```python
from build123d import *

# Parameters (mm, degrees)
SKETCH_R     = 3.375
PAD_DEPTH    = 3
SKETCH001_R  = 3.375
PAD001_DEPTH = 3
PAD002_DEPTH = 3
PAD003_DEPTH = 3
PAD004_DEPTH = 3


with BuildPart() as part:
    # Sketch → Pad (new body)
    with BuildSketch(Plane.XZ):
        with BuildLine():
            Line((-12.7, 0), (12.7, 0))
            Line((12.7, 0), (12.7, 52))
            ThreePointArc((12.7, 52), (0, 57.173882), (-12.7, 52))
            Line((-12.7, 52), (-12.7, 0))
        make_face()
        with Locations((0, 39)):
            Circle(SKETCH_R, mode=Mode.SUBTRACT)
        with Locations((0, 13)):
            Circle(SKETCH_R, mode=Mode.SUBTRACT)
    extrude(amount=-PAD_DEPTH)

    # Sketch001 → Pad001 (join)
    with BuildSketch(Plane.XY):
        with BuildLine():
            Line((-56.33961, 0), (-86.996465, 30.656854))
            ThreePointArc((-55.176659, 62.476659), (-78.231159, 53.711354), (-86.996465, 30.656854))
            Line((-55.176659, 62.476659), (4.3, 3))
            Line((4.3, 3), (-12.7, 3))
            Line((-12.7, 3), (-12.7, 0))
            Line((-56.33961, 0), (-12.7, 0))
        make_face()
        with Locations((-56.944426, 32.424621)):
            Circle(SKETCH001_R, mode=Mode.SUBTRACT)
    extrude(amount=PAD001_DEPTH)

    # Sketch002 → Pad002 (join)
    with BuildSketch(Plane.XZ):
        with BuildLine():
            Line((-12.7, 3), (-12.7, 52))
            ThreePointArc((-12.7, 52), (-14.569884, 49.487681), (-15.570964, 46.520182))
            ThreePointArc((-37.7, 3), (-23.321335, 23.074922), (-15.570964, 46.520182))
            Line((-12.7, 3), (-37.7, 3))
        make_face()
    extrude(amount=-PAD002_DEPTH)

    # Sketch003 → Pad003 (join)
    with BuildSketch(Plane.YZ.offset(-15)):
        Polygon((3, 3), (3, 33), (18, 3), align=None)
    extrude(amount=PAD003_DEPTH)

    # Sketch004 → Pad004 (join)
    with BuildSketch(Plane.YZ.offset(-25)):
        Polygon((3, 3), (3, 11), (11, 3), align=None)
    extrude(amount=-PAD004_DEPTH)


solid = part.part
```
Design review of the part built by this model. Coordinates are the model's own, in mm. A direction names the side the tool comes from. Coordinates: 2 decimals unless noted, no trailing zeros. Loops run counter-clockwise (first coordinate to the right, second up) from the corner with the lowest first, then second, coordinate; pieces in that order, holes last.
Q1. We need section B-B on z = 39. State the section outline as (x, y) points (3 decimals), and give its area (3 significant figures).
Reported:
outline: (-17.214, 0) - (-3.375, 0) - (-3.375, 3) - (-17.214, 3) - close; (3.375, 0) - (12.7, 0) - (12.7, 3) - (3.375, 3) - close
area: 69.5 mm2
Q2. We need section D-D on y = 7.5. State the section outline as (x, z) points, and give its area (3 significant figures).
Reported:
outline: (-63.84, 0) - (-0.2, 0) - (-0.2, 3) - (-12, 3) - (-12, 24) - (-15, 24) - (-15, 3) - (-25, 3) - (-25, 6.5) - (-28, 6.5) - (-28, 3) - (-63.84, 3) - close
area: 264 mm2
Q3. We need section C-C on z = 7. State the section outline as (x, y) points, and give its area (3 significant figures).
Reported:
outline: (-34.05, 0) - (12.7, 0) - (12.7, 3) - (-12, 3) - (-12, 16) - (-15, 16) - (-15, 3) - (-25, 3) - (-25, 7) - (-28, 7) - (-28, 3) - (-34.05, 3) - close
area: 191 mm2
Q4. To check wall thickness, follow line 1 (X direction, y = 6, z = 7); line 2 (Y direction, x = -14, z = 37). State the ranges of each line that lie inside material, in increasing order.
Reported:
line 1: x = -28 to -25, -15 to -12
line 2: y = 0 to 3
Q5. For pin 1 (12 mm diameter, centred on x = -30, z = 24.5, fed in from -Y); pin 2 (6.5 mm diameter, centred on y = 6.5, z = 8.5, fed in from -X); pin 3 (16.5 mm diameter, centred on y = 14, z = 13.5, fed in from -X), all flat-tipped, find the tip position at first contact; note any pin that passes through.
Reported:
pin 1: passes through
pin 2: stops at x = -28
pin 3: stops at x = -15
Q6. The part is to be moulded in two halves that separate along Z. For faces 4 (the face through (-14.549, 1.479, 49.527)), 5 (the face through (-77.98, 53.96, 1.48)), 6 (the face through (-0.439, 1.479, 16.346)), 7 (the face through (-0.7, 1.5, 35.7)), say which applies: +Z half, -Z half, draft (parallel to the pull), parting line (faces both ways), or undercut.
Reported:
face 4: +Z half
face 5: draft
face 6: undercut
face 7: undercut
Q7. Tool access review of faces 1 (the face through (-7, 3, 23)), 2 (the face through (-12, 7, 12)), 3 (the face through (-26, 7, 7)): name each direction out of +Z, -Z, +X, -X, +Y, -Y from which nothing blocks a thin tool from reaching the whole face with its end or side.
Reported:
face 1: +Z, +Y
face 2: +Z, +X, +Y
face 3: +Z, -X, +Y
Q8. We need section A-A on x = 0. State the section outline as (y, z) points (3 decimals), and give its area (3 significant figures).
Reported:
outline: (0, 0) - (7.3, 0) - (7.3, 3) - (3, 3) - (3, 9.625) - (0, 9.625) - close; (0, 16.375) - (3, 16.375) - (3, 35.625) - (0, 35.625) - close; (0, 42.375) - (3, 42.375) - (3, 57.174) - (0, 57.174) - close
area: 144 mm2
